```python
from build123d import *

# Parameters (mm, degrees)
F0_W     = 63.5
F0_H     = 38.1
F1_DEPTH = 127
F2_R     = 38.1
F3_DEPTH = 152.4
F4_SIZE  = 5.08
F6_D     = 76.2
F6_DEPTH = 38.101
F7_D     = 76.2


with BuildPart() as f1:
    # F0 (on Front) → F1 (new body)
    with BuildSketch(Plane.XZ):
        Polygon((137.8628114581, 133.5590133786), (99.7628114581, 133.5590133786), (99.7628114581, 95.4590133786), (99.7628114581, -69.6409866214), (137.8628114581, -69.6409866214), align=None)
        with Locations((68.0128114581, 114.5090133786)):
            Rectangle(F0_W, F0_H)
        with Locations((4.5128114581, 114.5090133786)):
            Rectangle(F0_W, F0_H)
        Polygon((-27.2371885419, 95.4590133786), (-27.2371885419, 133.5590133786), (-65.3371885419, 133.5590133786), (-65.3371885419, -69.6409866214), (-27.2371885419, -69.6409866214), align=None)
    extrude(amount=F1_DEPTH)

    # F2 (on face) → F3 (join)
    with BuildSketch(Plane.XY.offset(133.5590133786)):
        with Locations((36.2628114581, -63.5)):
            Circle(F2_R)
    extrude(amount=F3_DEPTH)

    # F4
    f4_edges = [f1.edges().sort_by_distance(p)[0] for p in [
        (-1.837189, -63.5, 285.959013),
    ]]
    chamfer(f4_edges, length=F4_SIZE)

    # F6 (through all, one way)
    with BuildSketch(Plane.YZ.offset(-27.2371885419)):
        with Locations((-63.5, 12.9090133786)):
            Circle(F6_D / 2)
    extrude(amount=-F6_DEPTH, mode=Mode.SUBTRACT)

    # F7 (through all)
    with Locations(Plane(origin=(-27.2371885419, 0, 0), x_dir=(0, 1, 0), z_dir=(-1, 0, 0))):
        with Locations((-63.5, -12.9090133786)):
            Hole(F7_D / 2)


solid = f1.part
```
Geometry: final body of the model. Coordinates: model frame, mm. A direction names the side the tool comes from. Coordinates: 2 decimals unless noted, no trailing zeros. Order: outer loops, then holes, each group sorted by start corner. A loop starts at its lowest first (then second) coordinate and runs counter-clockwise, first axis right, second up. Notation, with made-up numbers: (-12.75, -39) -> (6.25, -39) arc R23 ccw to (6.25, -29) -> close; hole circle Ø11 at (-25.5, 2.25). An arc over 180 degrees is marked (long way). Answer in a Markdown table with one row per item.
Item 1: Contact query for flat-ended pins moving along their axis: P1, Ø6, axis at y = -99.5, z = 178, coming from the +X side; P2, Ø5, axis at x = 43, y = -65, coming from the -Z side. Output: stop coordinate, or through.
Return value:
| item | result |
|---|---|
| P1 | stops at x = 55.31 |
| P2 | stops at z = 95.46 |
Item 2: Section A-A on y = -63.5. Output: boundary loops of the cut face in (x, z).
Return value:
| item | result |
|---|---|
| outline | (-65.34, -69.64) -> (-27.24, -69.64) -> (-27.24, -25.19) -> (-65.34, -25.19) -> close; (-65.34, 51.01) -> (-27.24, 51.01) -> (-27.24, 95.46) -> (99.76, 95.46) -> (99.76, 51.01) -> (137.86, 51.01) -> (137.86, 133.56) -> (74.36, 133.56) -> (74.36, 280.88) -> (69.28, 285.96) -> (3.24, 285.96) -> (-1.84, 280.88) -> (-1.84, 133.56) -> (-65.34, 133.56) -> close; (99.76, -69.64) -> (137.86, -69.64) -> (137.86, -25.19) -> (99.76, -25.19) -> close |
Item 3: Draft query along Z for faces 4 (the flat face through (137.863, -63, 53)), 5 (the flat face through (119, -63, -69.641)), 6 (the cylindrical face through (-46.02, -27.16, 24.35)). Return one class per face: released by +Z, released by -Z, zero draft, split by the parting line, or undercut.
Return value:
| item | result |
|---|---|
| face 4 | zero draft |
| face 5 | released by -Z |
| face 6 | undercut |
Item 4: Section D-D on y = -11. Output: boundary loops of the cut face in (x, z).
Return value:
| item | result |
|---|---|
| outline | (-65.34, -69.64) -> (-27.24, -69.64) -> (-27.24, 95.46) -> (99.76, 95.46) -> (99.76, -69.64) -> (137.86, -69.64) -> (137.86, 133.56) -> (-65.34, 133.56) -> close |
Item 5: Section B-B on z = 6. Output: boundary loops of the cut face in (x, y).
Return value:
| item | result |
|---|---|
| outline | (-65.34, -127) -> (-27.24, -127) -> (-27.24, -100.97) -> (-65.34, -100.97) -> close; (-65.34, -26.03) -> (-27.24, -26.03) -> (-27.24, 0) -> (-65.34, 0) -> close; (99.76, -127) -> (137.86, -127) -> (137.86, -100.97) -> (99.76, -100.97) -> close; (99.76, -26.03) -> (137.86, -26.03) -> (137.86, 0) -> (99.76, 0) -> close |
Item 6: Section C-C on x = -32.5. Output: boundary loops of the cut face in (y, z).
Return value:
| item | result |
|---|---|
| outline | (-127, -69.64) -> (0, -69.64) -> (0, 133.56) -> (-127, 133.56) -> close; hole circle Ø76.2 at (-63.5, 12.91) |
Item 7: Ray query, L1, parallel to Z at x = 118, y = -63.5; L2, parallel to X at y = -26, z = 32; L3, parallel to Z at x = -41, y = -22. Return the intervals inside material, ascending.
Return value:
| item | result |
|---|---|
| L1 | z = -69.64 to -25.19, 51.01 to 133.56 |
| L2 | x = -65.34 to -27.24, 99.76 to 137.86 |
| L3 | z = -69.64 to 133.56 |
Item 8: Access query for faces 1 (the flat face through (-65.337, -63, 56)), 2 (the cylindrical face through (72.603, -52.056, 206.188)), 3 (the flat face through (-27.237, -48, -25)). Directions: +Z, -Z, +X, -X, +Y, -Y. A direction counts if a zero-diameter tool reaches every point of the face in a straight line with its end or side. Return the directions, or none.
Return value:
| item | result |
|---|---|
| face 1 | +Z, -Z, -X, +Y, -Y |
| face 2 | +Z |
| face 3 | -Z, +Y, -Y |
